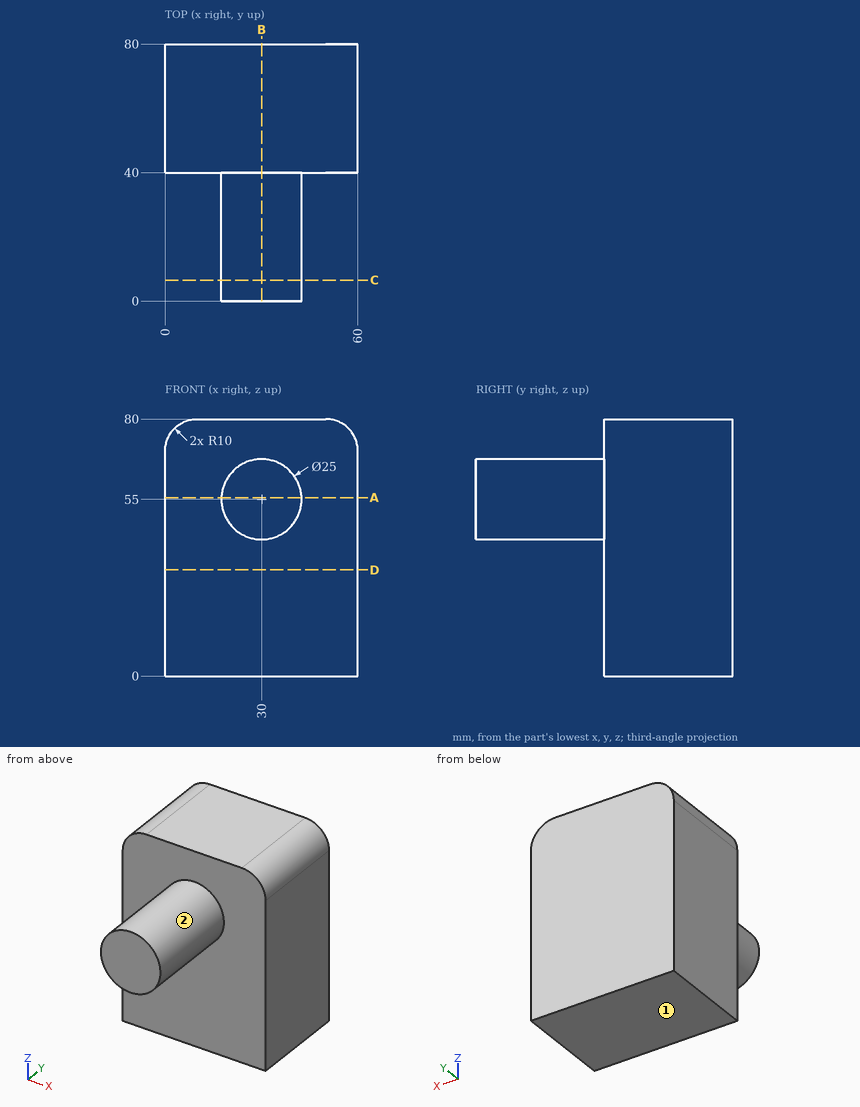
Here's the drawing with two shaded views (mm, measured from the low corner). I have some questions. A direction names the side the tool comes from. Round coordinates to 2 decimals unless told otherwise and drop trailing zeros. Order: outer loops, then holes, each group sorted by start corner. A loop starts at its lowest first (then second) coordinate and runs counter-clockwise, first axis right, second up. Notation, with made-up numbers: (66.5, 48) -> (123.5, 48) arc R23 cw to (123.5, 69) -> close; hole circle Ø2 at (25, -24.5). An arc over 180 degrees is marked (long way). Return JSON: item names as keys, results as strings.
Q1. If we section it at D-D on z = 33: List the corners of the cut face in (x, y) for me.
Filled sheet:
{"outline": "(0, 40) -> (60, 40) -> (60, 80) -> (0, 80) -> close"}
Q2. Which directions (+Z, -Z, +X, -X, +Y, -Y) give clear straight access to the entire face, cutting with the end or side of a thin tool? Please do the marked faces 1 and 2.
Filled sheet:
{"face 1": "-Z, +X, -X, +Y, -Y", "face 2": "-Y"}
Q3. If we section it at B-B on x = 30: List the corners of the cut face in (y, z) for me.
Filled sheet:
{"outline": "(0, 42.5) -> (40, 42.5) -> (40, 0) -> (80, 0) -> (80, 80) -> (40, 80) -> (40, 67.5) -> (0, 67.5) -> close"}
Q4. For pin 1 Ø10 at (x, y) = (19.5, 30) entering from -Z (3 decimals); pin 2 Ø1.5 at (x, y) = (21.5, 22.5) entering from -Z; pin 3 Ø8 at (x, y) = (44, 11) entering from -Z, each with a flat end and sliding along its axis, tell me the tip position at first contact or that it passes through.
Filled sheet:
{"pin 1": "stops at z = 43.775", "pin 2": "stops at z = 45.19", "pin 3": "stops at z = 47.5"}
Q5. I need wall thicknesses on line 1 along Y through (x, z) = (41.5, 69.5); line 2 along Z through (x, y) = (9.5, 56.5); line 3 along Z through (x, y) = (4, 49). Which ranges of each line are inside material? Lowest first, please. Write a range as from..to.
Filled sheet:
{"line 1": "y = 40..80", "line 2": "z = 0..79.99", "line 3": "z = 0..78"}
Q6. If we section it at C-C on y = 6.5: List the corners of the cut face in (x, z) for me, plus the area to 3 significant figures.
Filled sheet:
{"outline": "circle Ø25 at (30, 55)", "area": "491 mm^2"}
Q7. If we section it at A-A on z = 55.5: List the corners of the cut face in (x, y) for me.
Filled sheet:
{"outline": "(0, 40) -> (17.51, 40) -> (17.51, 0) -> (42.49, 0) -> (42.49, 40) -> (60, 40) -> (60, 80) -> (0, 80) -> close"}
